Can you work these out from the model? Positions are in its coordinate system, mm. Face numbers are marked on the shaded views. A direction names the side the tool comes from. Give positions to 0.01 mm unless a question says otherwise; leave off trailing zeros. Write each loop counter-clockwise with the first axis right and the second up, starting at its lowest first coordinate (ties: lowest second). Pieces come first, ordered by that corner, then holes. Notation, with made-up numbers: (67.25, 29.5) - (126.25, 29.5) arc R8 cw to (126.25, 44.5) - close; hole circle Ø8 at (52, 52). An arc over 180 degrees is marked (long way). Use a Markdown table: item, result. Add a question column.
```python
from build123d import *

# Parameters (mm, degrees)
F0_W     = 108.5
F0_H     = 61.5
F0_W_2   = 85.5
F0_H_2   = 45.5
F1_DEPTH = 3
F2_W     = 3
F2_H     = 15
F3_DEPTH = 1.7
F4_W     = 108.5
F4_H     = 61.5
F4_W_2   = 104.5
F4_H_2   = 57.5
F5_DEPTH = 22
F7_DEPTH = 2


with BuildPart() as f1:
    # F0 (on Top) → F1 (new body)
    with BuildSketch(Plane.XY):
        with Locations((39.25, 22.75)):
            Rectangle(F0_W, F0_H)
        with Locations((42.75, 22.75)):
            Rectangle(F0_W_2, F0_H_2, mode=Mode.SUBTRACT)
    extrude(amount=F1_DEPTH)

    # F2 (on face) → F3 (cut, through all)
    with BuildSketch(Plane.XY.offset(3)):
        with Locations((-1.5, 23)):
            Rectangle(F2_W, F2_H)
        with Locations((87, 23)):
            Rectangle(F2_W, F2_H)
    extrude(amount=-F3_DEPTH, mode=Mode.SUBTRACT)

    # F4 (on face) → F5 (join)
    with BuildSketch(Plane.XY.offset(3)):
        with Locations((39.25, 22.75)):
            Rectangle(F4_W, F4_H)
        with Locations((39.25, 22.75)):
            Rectangle(F4_W_2, F4_H_2, mode=Mode.SUBTRACT)
    extrude(amount=F5_DEPTH)

    # F6 (on face) → F7 (cut, through all)
    with BuildSketch(Plane(origin=(0, 53.5, 0), x_dir=(-1, 0, 0), z_dir=(0, 1, 0))):
        with BuildLine():
            Line((11, 25), (6.1561632305, 25))
            ThreePointArc((6.1561632305, 25), (8.5780816153, 22.5780816153), (11, 25))
        make_face()
    extrude(amount=-F7_DEPTH, mode=Mode.SUBTRACT)


solid = f1.part
```
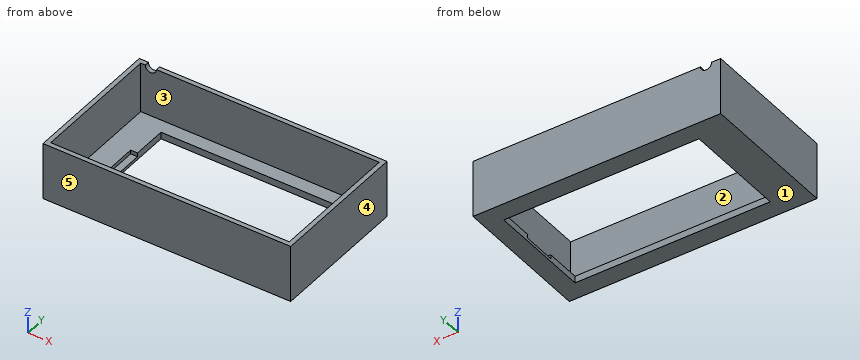
Q1. If we mould it in two halves opening along X, with no side actions, what happens to the marked faces 3, 4 and 5? For each: released by +X, released by -X, zero draft, split by the parting line, or undercut.
Q2. I'm going to push a flat-ended pin straight in: P1, Ø0.9, axis at x = -1, y = 24.5, coming from the +Z side. Where does the tip first touch, or does it pass through?
Q3. Suppose I cut it at C-C (x = 45). Please give me the cut outline in (y, z), and give its area (3 significant figures).
Q4. On a 3-axis mill with a long thin cutter (end or side, diameter ignored), from which of +Z, -Z, +X, -X, +Y, -Y can I reach the whole of each face in a straight line? I mean the marked faces 1 and 2. Say none if no direction works.
Q5. Suppose I cut it at D-D (y = 34). Please give me the cut outline in (x, z), and give its area (3 significant figures).
Q6. Suppose I cut it at A-A (y = 18.5). Please give me the cut outline in (x, z), and give its area (3 significant figures).
Q7. Suppose I cut it at B-B (z = 17). Please give me the cut outline in (x, y).
Q8. If I drill on probe 1 along Y at (x, z) = (38, 21); probe 2 along X at (y, z) = (10, 17.25); probe 3 along Z at (x, y) = (86, 11.5), over which ranges is the centre line in solid material (lowest first)? Write a range as [from, to].
Derived:
| question | item | result |
|---|---|---|
| 1 | face 3 | undercut |
| 1 | face 4 | released by +X |
| 1 | face 5 | zero draft |
| 2 | P1 | z = 1.3 |
| 3 | outline | (-8, 0) - (0, 0) - (0, 3) - (-6, 3) - (-6, 25) - (-8, 25) - close; (45.5, 0) - (53.5, 0) - (53.5, 25) - (51.5, 25) - (51.5, 3) - (45.5, 3) - close |
| 3 | area | 136 mm² |
| 4 | face 1 | -Z, +X, -X, +Y, -Y |
| 4 | face 2 | +Z |
| 5 | outline | (-15, 0) - (0, 0) - (0, 3) - (-13, 3) - (-13, 25) - (-15, 25) - close; (85.5, 0) - (93.5, 0) - (93.5, 25) - (91.5, 25) - (91.5, 3) - (85.5, 3) - close |
| 5 | area | 157 mm² |
| 6 | outline | (-15, 0) - (0, 0) - (0, 1.3) - (-3, 1.3) - (-3, 3) - (-13, 3) - (-13, 25) - (-15, 25) - close; (85.5, 0) - (93.5, 0) - (93.5, 25) - (91.5, 25) - (91.5, 3) - (88.5, 3) - (88.5, 1.3) - (85.5, 1.3) - close |
| 6 | area | 147 mm² |
| 7 | outline | (-15, -8) - (93.5, -8) - (93.5, 53.5) - (-15, 53.5) - close; hole (-13, -6) - (91.5, -6) - (91.5, 51.5) - (-13, 51.5) - close |
| 8 | probe 1 | [-8, -6], [51.5, 53.5] |
| 8 | probe 2 | [-15, -13], [91.5, 93.5] |
| 8 | probe 3 | [0, 3] |
